```python
from build123d import *

# Parameters (mm, degrees)
CHAMFER1_SIZE      = 0.35
CUT_EXTRUDE1_START = -1.8000001
CUT_EXTRUDE1_DEPTH = 2.8000001
FILLET1_R          = 0.2


with BuildPart() as part:
    # Sketch1 → Revolve1 (revolve)
    with BuildSketch(Plane(origin=(0, 0, 0), x_dir=(0, 0, -1), z_dir=(1, 0, 0)), mode=Mode.PRIVATE) as revolve1_sk:
        with BuildLine():
            Line((10, 0), (10, 2))
            Line((10, 2), (0, 2))
            Line((0, 2), (0, 3.75))
            Line((0, 3.75), (-0.4, 3.75))
            ThreePointArc((-0.4, 3.75), (-1.845304899, 3.217657748), (-2.6, 1.875))
            Line((-2.6, 1.875), (-2.6, 0))
            Line((-2.6, 0), (10, 0))
        make_face()
    revolve(revolve1_sk.sketch.rotate(Axis((0, 0, 30.809969789), (0, 0, -1)), 90), axis=Axis((0, 0, 30.809969789), (0, 0, -1)))

    # Chamfer1
    chamfer1_edges = [part.edges().sort_by_distance(p)[0] for p in [
        (-2, 0, -10),
    ]]
    chamfer(chamfer1_edges, length=CHAMFER1_SIZE)

    # Sketch2 → Cut-Revolve1 (revolve, cut)
    with BuildSketch(Plane(origin=(0, 0, 0), x_dir=(0, 0, -1), z_dir=(1, 0, 0)), mode=Mode.PRIVATE) as cut_revolve1_sk:
        Polygon((-2.6, 0), (-2.6, 1.25), (-0.8, 1.25), (-0.078312164, 0), align=None)
    revolve(cut_revolve1_sk.sketch.rotate(Axis((0, 0, 2.452500839), (0, 0, -1)), 90), axis=Axis((0, 0, 2.452500839), (0, 0, -1)), mode=Mode.SUBTRACT)

    # Cut-Extrude1: read off the stored shape, not the designer's step
    # Cut-Extrude1 outline → Cut-Extrude1 (cut)
    with BuildSketch(Plane.XY.offset(2.6).offset(CUT_EXTRUDE1_START)):
        with BuildLine():
            Line((1.25, 0), (1.25, 0.721687836))
            Line((1.25, 0.721687836), (0.625, 1.082531755))
            ThreePointArc((0.625, 1.082531755), (1.082531755, 0.625), (1.25, 0))
        make_face()
        with BuildLine():
            ThreePointArc((-0.625, 1.082531755), (0, 1.25), (0.625, 1.082531755))
            Line((0.625, 1.082531755), (0, 1.443375673))
            Line((0, 1.443375673), (-0.625, 1.082531755))
        make_face()
        with BuildLine():
            Line((1.25, -0.721687836), (1.25, 0))
            ThreePointArc((1.25, 0), (1.082531755, -0.625), (0.625, -1.082531755))
            Line((0.625, -1.082531755), (1.25, -0.721687836))
        make_face()
        with BuildLine():
            ThreePointArc((-1.25, 0), (-1.082531755, 0.625), (-0.625, 1.082531755))
            Line((-0.625, 1.082531755), (-1.25, 0.721687836))
            Line((-1.25, 0.721687836), (-1.25, 0))
        make_face()
        with BuildLine():
            Line((0, -1.443375673), (0.625, -1.082531755))
            ThreePointArc((0.625, -1.082531755), (0, -1.25), (-0.625, -1.082531755))
            Line((-0.625, -1.082531755), (0, -1.443375673))
        make_face()
        with BuildLine():
            ThreePointArc((-0.625, -1.082531755), (-1.082531755, -0.625), (-1.25, 0))
            Line((-1.25, 0), (-1.25, -0.721687836))
            Line((-1.25, -0.721687836), (-0.625, -1.082531755))
        make_face()
    extrude(amount=CUT_EXTRUDE1_DEPTH, mode=Mode.SUBTRACT)

    # Cut-Extrude1 2 outline → Cut-Extrude1 2 (revolve)
    with BuildSketch(Plane.XZ):
        Polygon((1.443375738, 0.911645534), (1.249999957, 0.799999975), (1.443375673, 0.7999999), align=None)
    revolve(axis=Axis((0, 0, 0), (0, 0, 1)))

    # Fillet1
    fillet1_edges = [part.edges().sort_by_distance(p)[0] for p in [
        (-2, 0, 0),
    ]]
    fillet(fillet1_edges, radius=FILLET1_R)


solid = part.part
```
Geometry check sheet. Reference: the model listing, model coordinates, mm. A direction names the side the tool comes from. Coordinates: 2 decimals unless noted, no trailing zeros. Loops run counter-clockwise (first coordinate to the right, second up) from the corner with the lowest first, then second, coordinate; pieces in that order, holes last. Notation, with made-up numbers: (-17.75, 68) -> (27.25, 68) arc R23 ccw to (27.25, 101) -> close; hole circle Ø11 at (-17.5, 25). An arc over 180 degrees is marked (long way). Put each result on its own line as item: value.
1) Cross-section at A-A on z = -3.5. Record the boundary of the cut face in (x, y), plus the area to 3 significant figures.
Result set:
outline: circle Ø4 at (0, 0)
area: 12.6 mm^2
2) Release check for a two-part mould opening along X. For faces 3 (the flat face through (-2, 2, 0)), 4 (the cylindrical face through (0, 2, -5)), 5 (the flat face through (1.25, 0, 2)) record: released by +X, released by -X, zero draft, split by the parting line, or undercut.
Result set:
face 3: zero draft
face 4: split by the parting line
face 5: undercut
3) Gauge pin test, flat ends, axial feed: pin 1 Ø2 at (x, z) = (2.5, -2.5) entering from +Y; pin 2 Ø0.7 at (y, z) = (0, 1.5) entering from -X; pin 3 Ø1 at (x, z) = (0.5, -3) entering from -Y. Record the tip position at first contact, or that the pin passes through.
Result set:
pin 1: stops at y = 1.32
pin 2: stops at x = -3.62
pin 3: stops at y = -2
4) Tool access check on faces 1 (the flat face through (-1.25, 0, 2)), 2 (the flat face through (0, 0, -10)). Record the directions out of +Z, -Z, +X, -X, +Y, -Y that give a thin tool (end or side, any length) a straight path to the whole face; none if there is none.
Result set:
face 1: +Z
face 2: -Z, +X, -X, +Y, -Y
5) Thickness scan on line 1 (Z direction, x = -0.75, y = -3); line 2 (Z direction, x = -3, y = -1); line 3 (Y direction, x = -1, z = -7). Record the ranges inside material, lowest first.
Result set:
line 1: z = 0 to 1.98
line 2: z = 0 to 1.91
line 3: y = -1.73 to 1.73
